Can you work these out from the model? Positions are in its coordinate system, mm. A direction names the side the tool comes from. Give positions to 0.01 mm unless a question says otherwise; leave off trailing zeros. Order: outer loops, then holes, each group sorted by start corner. A loop starts at its lowest first (then second) coordinate and runs counter-clockwise, first axis right, second up. Notation, with made-up numbers: M 40.5,21.5 L 52.5,21.5 A36 ccw 52.5,57.5 Z; hole C -22.75,42 d7. An arc over 180 degrees is marked long. One line per question, with ' | ' between items. Start each with the question number.
1) I'm going to push flat-ended pins straight in: pin 1 Ø2 at (x, y) = (-5, -8) entering from -Z; pin 2 Ø2 at (x, y) = (-9, 3) entering from -Z; pin 3 Ø7.5 at (x, z) = (-14, 2) entering from -Y. Where does each tip first touch, or does it pass through?
2) For faces 5 (the flat face through (3.215, 0.056, 12)), 6 (the flat face through (6, -4, 11)), 7 (the cylindrical face through (-1.08, 11.55, 4.88)), 8 (the flat face through (0, 15, 0)), which set-ups out of +Z, -Z, +X, -X, +Y, -Y let a thin tool reach every point of the face, with its end or its side?
3) If we section it at C-C, the plane y = -6.5: Please give me the cut outline in (x, z).
4) If we section it at A-A, the plane x = 0: State how many separate pieces and enclosed holes the cut face has, plus the area to 3 significant figures.
5) Thinking about a two-plate mould opening in X: for faces 1 (the flat face through (-5, 8, -2)), 2 (the flat face through (12.148, 0.056, -3.255)), 3 (the cylindrical face through (-29.97, 0.03, -1.32)), 4 (the flat face through (6, 4, 11)), which applies, +X half, -X half, draft (parallel to the pull), parting line (faces both ways), or undercut?
6) Please list where these lines run through material, in increasing order: line 1 along X through (y, z) = (-5.55, 0); line 2 along Z through (x, y) = (0, 7); line 3 along X through (y, z) = (-5.5, 0). Write a range as [from, to].
```python
from build123d import *

# Parameters (mm, degrees)
SKETCH_1_R               = 5
EXTRUDE_1_DEPTH          = 15
EXTRUDE_1_DEPTH_BACK     = 15
SKETCH_2_R               = 20
EXTRUDE_2_DEPTH          = 8
EXTRUDE_2_DEPTH_BACK     = 8
SKETCH_4_R               = 18
SKETCH_4_R_2             = 7
CUT_EXTRUDE_1_DEPTH      = 4
CUT_EXTRUDE_2_DEPTH      = 14
PATTERN_CIRCULAR_1_COUNT = 6
SKETCH_6_R               = 30
SKETCH_6_R_2             = 20
EXTRUDE_3_DEPTH          = 7.99
EXTRUDE_3_DEPTH_BACK     = 7.99
FILLET_1_R               = 6


with BuildPart() as part:
    # Sketch 1 → Extrude 1 (new body, two sides)
    with BuildSketch(Plane(origin=(0, 0, 0), x_dir=(1, 0, 0), z_dir=(0, 1, 0))) as extrude_1_sk:
        Circle(SKETCH_1_R)
    extrude(amount=EXTRUDE_1_DEPTH)
    extrude(extrude_1_sk.sketch, amount=-EXTRUDE_1_DEPTH_BACK)

    # Sketch 2 → Extrude 2 (add, two sides)
    with BuildSketch(Plane(origin=(0, 0, 0), x_dir=(1, 0, 0), z_dir=(0, 1, 0))) as extrude_2_sk:
        Circle(SKETCH_2_R)
    extrude(amount=EXTRUDE_2_DEPTH)
    extrude(extrude_2_sk.sketch, amount=-EXTRUDE_2_DEPTH_BACK)

    # Sketch 4 → Cut-Extrude 1 (cut)
    with BuildSketch(Plane(origin=(0, 8, 0), x_dir=(1, 0, 0), z_dir=(0, 1, 0))):
        Circle(SKETCH_4_R)
        Circle(SKETCH_4_R_2, mode=Mode.SUBTRACT)
    cut_extrude_1 = extrude(amount=-CUT_EXTRUDE_1_DEPTH, mode=Mode.SUBTRACT)

    # Mirror 1: Cut-Extrude 1 across plane
    add(cut_extrude_1.mirror(Plane.ZX), mode=Mode.SUBTRACT)

    # Sketch 5 → Cut-Extrude 2 (cut)
    with BuildSketch(Plane(origin=(0, 4, 0), x_dir=(1, 0, 0), z_dir=(0, 1, 0))):
        with BuildLine():
            Line((-1.811733, 6.761481), (-4.658743, 17.386665))
            ThreePointArc((-4.658743, 17.386665), (0, 18), (4.658743, 17.386665))
            Line((4.658743, 17.386665), (1.811733, 6.761481))
            ThreePointArc((1.811733, 6.761481), (0, 7), (-1.811733, 6.761481))
        make_face()
    cut_extrude_2 = extrude(amount=-CUT_EXTRUDE_2_DEPTH, mode=Mode.SUBTRACT)

    # Pattern Circular 1: Cut-Extrude 2 ×6 about axis
    pattern_circular_1_axis = Axis((0, 0, 0), (0, 1, 0))
    for i in range(1, PATTERN_CIRCULAR_1_COUNT):
        add(cut_extrude_2.rotate(pattern_circular_1_axis, i * 360 / PATTERN_CIRCULAR_1_COUNT), mode=Mode.SUBTRACT)

    # Sketch 6 → Extrude 3 (add, two sides)
    with BuildSketch(Plane(origin=(0, 0, 0), x_dir=(1, 0, 0), z_dir=(0, 1, 0))) as extrude_3_sk:
        Circle(SKETCH_6_R)
        Circle(SKETCH_6_R_2, mode=Mode.SUBTRACT)
    extrude(amount=EXTRUDE_3_DEPTH)
    extrude(extrude_3_sk.sketch, amount=-EXTRUDE_3_DEPTH_BACK)

    # Fillet 1
    fillet_1_edges = [part.edges().sort_by_distance(p)[0] for p in [
        (-30, -7.99, 0),
        (-30, 7.99, 0),
    ]]
    fillet(fillet_1_edges, radius=FILLET_1_R)


solid = part.part
```
Results found:
1) pin 1: stops at z = -26.85 | pin 2: stops at z = -28.86 | pin 3: stops at y = -4
2) face 5: +Y, -Y | face 6: -Y | face 7: +Y | face 8: +Z, -Z, +X, -X, +Y
3) outline: C 0,0 d55.91; C 0,0 d14; hole C 0,0 d36
4) separate pieces: 3 | enclosed holes: 0 | area: 717 mm²
5) face 1: draft | face 2: undercut | face 3: parting line | face 4: undercut
6) line 1: x = [-28.83, -18], [-7, 7], [18, 28.83] | line 2: z = [-27.3, -18], [-7, 7], [18, 27.3] | line 3: x = [-28.87, -18], [-7, 7], [18, 28.87]
